from build123d import *

# Parameters (mm, degrees)
SKETCH_1_W            = 24
SKETCH_1_H            = 18
EXTRUDE_1_DEPTH       = 10
SKETCH_2_R            = 9
SKETCH_2_R_2          = 5.275
EXTRUDE_2_DEPTH       = 6
SKETCH_3_R            = 2.55
CUT_EXTRUDE_1_DEPTH   = 41
SKETCH_4_R            = 1.55
CUT_EXTRUDE_2_DEPTH   = 37.013519789
M4_TAPPED_HOLE1_D     = 3.3
M4_TAPPED_HOLE1_DEPTH = 23.5
M4_TAPPED_HOLE1_TIP   = 0.991420021
SKETCH2_R             = 7.475
SKETCH2_R_2           = 5.275
BOSS_EXTRUDE1_DEPTH   = 6
CHAMFER1_SIZE         = 0.5
SKETCH3_R             = 5
CUT_EXTRUDE1_DEPTH    = 5
FILLET1_R             = 3


with BuildPart() as part:
    # 草图1 → 凸台-拉伸1 (new body)
    with BuildSketch(Plane.XY):
        Rectangle(SKETCH_1_W, SKETCH_1_H)
    extrude(amount=EXTRUDE_1_DEPTH)

    # 草图2 → 凸台-拉伸2 (add)
    with BuildSketch(Plane.XY):
        Circle(SKETCH_2_R)
        Circle(SKETCH_2_R_2, mode=Mode.SUBTRACT)
    extrude(amount=-EXTRUDE_2_DEPTH)

    # 草图3 → 切除-拉伸1 (cut)
    with BuildSketch(Plane(origin=(0, 0, 0), x_dir=(-1, 0, 0), z_dir=(0, 0, -1))):
        Circle(SKETCH_3_R)
    extrude(amount=-CUT_EXTRUDE_1_DEPTH, mode=Mode.SUBTRACT)

    # 草图4 → 切除-拉伸2 (cut)
    with BuildSketch(Plane(origin=(0, 9, 0), x_dir=(1, 0, 0), z_dir=(0, 1, 0))):
        with Locations(Location((-8, -5, 0), (0, 0, 270))):
            Circle(SKETCH_4_R)
        with Locations(Location((8, -5, 0), (0, 0, 270))):
            Circle(SKETCH_4_R)
    extrude(amount=-CUT_EXTRUDE_2_DEPTH, mode=Mode.SUBTRACT)

    # M4 Tapped Hole1
    with Locations(Plane(origin=(9, 0, 0), x_dir=(0, 0, -1), z_dir=(1, 0, 0))):
        with Locations((3, 0)):
            Hole(M4_TAPPED_HOLE1_D / 2, depth=M4_TAPPED_HOLE1_DEPTH)
            with Locations((0, 0, -(M4_TAPPED_HOLE1_DEPTH + M4_TAPPED_HOLE1_TIP / 2))):  # 118° drill point
                Cone(0, M4_TAPPED_HOLE1_D / 2, M4_TAPPED_HOLE1_TIP, mode=Mode.SUBTRACT)

    # Sketch2 → Boss-Extrude1 (add)
    with BuildSketch(Plane(origin=(0, 0, -6), x_dir=(-1, 0, 0), z_dir=(0, 0, -1))):
        Circle(SKETCH2_R)
        with Locations(Location((0, 0, 0), (0, 0, 180))):
            Circle(SKETCH2_R_2, mode=Mode.SUBTRACT)
    extrude(amount=BOSS_EXTRUDE1_DEPTH)

    # Chamfer1
    chamfer1_edges = [part.edges().sort_by_distance(p)[0] for p in [
        (-9, 0, -6),
        (7.475, 0, -12),
    ]]
    chamfer(chamfer1_edges, length=CHAMFER1_SIZE)

    # Sketch3 → Cut-Extrude1 (cut)
    with BuildSketch(Plane.XY.offset(10)):
        Circle(SKETCH3_R)
    extrude(amount=-CUT_EXTRUDE1_DEPTH, mode=Mode.SUBTRACT)

    # Fillet1
    fillet1_edges = [part.edges().sort_by_distance(p)[0] for p in [
        (-12, 0, 10),
        (12, 0, 10),
        (-12, 0, 0),
        (12, 0, 0),
    ]]
    fillet(fillet1_edges, radius=FILLET1_R - 0.0001)  # a hair under: the kernel refuses the full size


solid = part.part
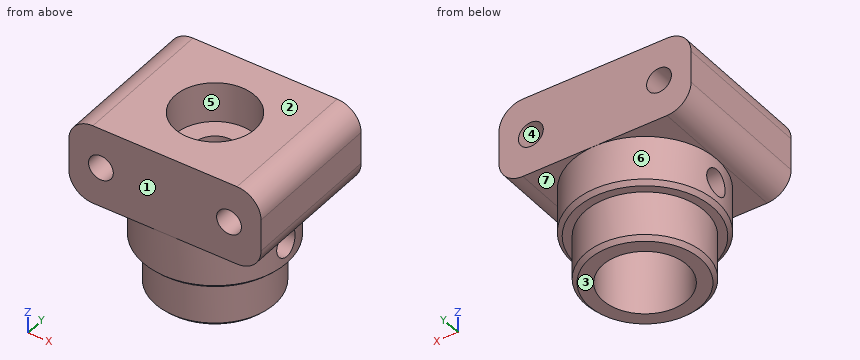
Read the model definition and answer for the solid it produces. Units are mm, in the model's axes. Face numbers are marked on the shaded views. A direction names the side the tool comes from. Give positions to 0.01 mm unless a question says otherwise; leave off trailing zeros. Write each loop counter-clockwise with the first axis right and the second up, starting at its lowest first coordinate (ties: lowest second). Pieces come first, ordered by that corner, then holes. Notation, with made-up numbers: (-19, 85) - (16, 85) arc R14 cw to (16, 106) - close; hole circle Ø3 at (-4, -17.5). An arc over 180 degrees is marked (long way). Use CSV: the item, a comma, the result in double quotes. Start each with the question number.
Item 1: The mould has two halves that part along Z. Classify the marked faces 1, 2, 3 and 4: pulls with the +Z half, pulls with the -Z half, needs draft (parallel to the pull), parting line crosses it, or undercut.
Item 2: The part is cut by section C-C, the plane y = 0. Count the separate pieces of the cut face and the enclosed holes in it, and give its area (3 significant figures).
Item 3: The part is cut by section A-A, the plane z = 4. Give the vertices of the cut face in (x, y).
Item 4: Consider line 1 (Y direction, x = 0, z = -4.25) (3 decimals); line 2 (Z direction, x = -7.2, y = 0) (3 decimals); line 3 (Z direction, x = 8.25, y = -1.25). Determine where each line is inside the solid, lowest interval first.
Item 5: The part is cut by section B-B, the plane z = -3. Give the vertices of the cut face in (x, y) (3 decimals), and give its area (3 significant figures).
Item 6: For the marked faces 5, 6 and 7, determine the directions among +Z, -Z, +X, -X, +Y, -Y from which every point of the face is accessible in a straight line to the end or side of a thin tool.
Item 7: Flat-ended cylindrical pins translate along their axes: P1, Ø4.5, axis at y = 0, z = -3, coming from the -X side; P2, Ø3, axis at x = 2.5, y = 1.5, coming from the -Z side; P3, Ø5, axis at y = -5.5, z = -1, coming from the +X side. Find the tip coordinate at first contact, or state that the pin passes through.
Taken from the geometry:
1,face 1,"needs draft"
1,face 2,"pulls with the +Z half"
1,face 3,"pulls with the -Z half"
1,face 4,"undercut"
2,separate pieces,"4"
2,enclosed holes,"2"
2,area,"188 mm2"
3,outline,"(-12, -9) - (-9.18, -9) - (-9.18, 9) - (-12, 9) - close; (-6.82, -9) - (6.82, -9) - (6.82, 9) - (-6.82, 9) - close; (9.18, -9) - (12, -9) - (12, 9) - (9.18, 9) - close; hole circle Ø5.1 at (0, 0)"
4,line 1,"-9 to -5.275, 5.275 to 9"
4,line 2,"-11.775 to -4.65, -1.35 to 3.672, 6.328 to 10"
4,line 3,"-6 to -4.08, -1.92 to 3.47, 6.53 to 10"
5,outline,"(-8.847, -1.65) arc R9 ccw to (8.847, -1.65) - (5.01, -1.65) arc R5.275 cw to (-5.01, -1.65) - close; (-8.847, 1.65) - (-5.01, 1.65) arc R5.275 cw to (5.01, 1.65) - (8.847, 1.65) arc R9 ccw to start"
5,area,"142 mm2"
6,face 5,"+Z"
6,face 6,"-Z"
6,face 7,"-Z, +X"
7,P1,"x = -9"
7,P2,"z = 0"
7,P3,"x = 11.6"
